from build123d import *

# Parameters (mm, degrees)
BOSS_EXTRU_1_DEPTH      = 21
ENL_V_MAT_EXTRU_1_REACH = 33.267
ESQUISSE2_R             = 3
ESQUISSE3_R             = 6
ENL_V_MAT_EXTRU_2_DEPTH = 10


with BuildPart() as part:
    # Esquisse1 → Boss.-Extru.1 (new body)
    with BuildSketch(Plane(origin=(0, 0, 0), x_dir=(0, 0, -1), z_dir=(1, 0, 0))):
        with BuildLine():
            Line((-42, -117.732748205), (-42, -149))
            Line((-42, -149), (42, -149))
            Line((42, -149), (42, -117.732748205))
            ThreePointArc((42, -117.732748205), (0, -125), (-42, -117.732748205))
        make_face()
    extrude(amount=BOSS_EXTRU_1_DEPTH)

    # Esquisse2 → Enlèv. mat.-Extru.1 (cut, up to next)
    with BuildSketch(Plane.XZ.offset(149), mode=Mode.PRIVATE) as enl_v_mat_extru_1_sk1:
        with Locations((10.5, 0)):
            Circle(ESQUISSE2_R)
    enl_v_mat_extru_1_tool1 = extrude(enl_v_mat_extru_1_sk1.sketch, amount=-ENL_V_MAT_EXTRU_1_REACH, mode=Mode.PRIVATE) & part.part
    add(enl_v_mat_extru_1_tool1.solids().sort_by_distance((10.5, -149, 0))[0], mode=Mode.SUBTRACT)

    # Esquisse3 → Enlèv. mat.-Extru.2 (cut)
    with BuildSketch(Plane.XZ.offset(149)):
        with Locations((10.560210211, 0)):
            Circle(ESQUISSE3_R)
    extrude(amount=-ENL_V_MAT_EXTRU_2_DEPTH, mode=Mode.SUBTRACT)


solid = part.part
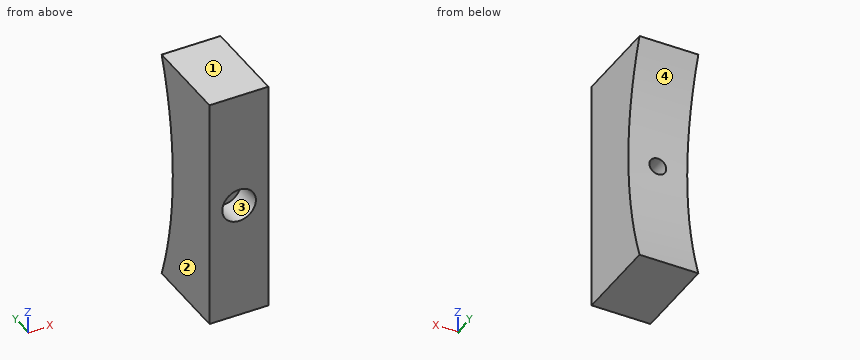
Geometry check sheet. Reference: the model listing, model coordinates, mm. Face numbers are marked on the shaded views. Give positions to 0.01 mm unless a question says otherwise; leave off trailing zeros. Order: outer loops, then holes, each group sorted by start corner. A loop starts at its lowest first (then second) coordinate and runs counter-clockwise, first axis right, second up. Notation, with made-up numbers: M -26.75,-19 L -15.75,-19 A11 ccw -15.75,-9 Z; hole C 20,25 d6. An arc over 180 degrees is marked long. Use a Markdown table: item, result.
Item 1: Section check D-D (x = 18.5). Record the cut outline in (y, z).
Answers follow:
| item | result |
|---|---|
| outline | M -149,-42 L -117.73,-42 A125 cw -117.73,42 L -149,42 Z |
Item 2: Material ranges on line 1 along X through (y, z) = (-131.75, 0); line 2 along Z through (x, y) = (10.5, -130.5); line 3 along Z through (x, y) = (13.75, -141.5), recorded low to high.
Answers follow:
| item | result |
|---|---|
| line 1 | x = 0 to 7.5, 13.5 to 21 |
| line 2 | z = -42 to -3, 3 to 42 |
| line 3 | z = -42 to -5.08, 5.08 to 42 |
Item 3: Section check B-B (x = 12). Record the cut outline in (y, z), and give its area (3 significant figures).
Answers follow:
| item | result |
|---|---|
| outline | M -149,-42 L -117.73,-42 A125 cw -124.97,-2.6 L -139,-2.6 L -139,-5.82 L -149,-5.82 Z; M -149,5.82 L -139,5.82 L -139,2.6 L -124.97,2.6 A125 cw -117.73,42 L -149,42 Z |
| area | 2,030 mm2 |
Item 4: Depth check by flat-ended pin: P1, Ø1, axis at x = 4.5, z = -18, coming from the +Y side; P2, Ø6, axis at x = 12.5, z = -2, coming from the -Y side; P3, Ø3, axis at x = 18.5, z = -1, coming from the +Y side (3 decimals); P4, Ø4, axis at y = -130.5, z = 16.5, coming from the -X side. Enter the tip coordinate at first touch or a pass-through.
Answers follow:
| item | result |
|---|---|
| P1 | stops at y = -123.62 |
| P2 | stops at y = -139 |
| P3 | stops at y = -124.975 |
| P4 | stops at x = 0 |
Item 5: Section check A-A (z = 0). Record the cut outline in (x, y).
Answers follow:
| item | result |
|---|---|
| outline | M 0,-149 L 4.56,-149 L 4.56,-139 L 7.5,-139 L 7.5,-125 L 0,-125 Z; M 13.5,-139 L 16.56,-139 L 16.56,-149 L 21,-149 L 21,-125 L 13.5,-125 Z |
Item 6: Draft check along Z on the marked faces 1, 2, 3 and 4. Enter one of: +Z half, -Z half, draft (parallel to the pull), parting line (faces both ways), or undercut.
Answers follow:
| item | result |
|---|---|
| face 1 | +Z half |
| face 2 | draft |
| face 3 | undercut |
| face 4 | undercut |
Item 7: Section check C-C (y = -137). Record the cut outline in (x, z).
Answers follow:
| item | result |
|---|---|
| outline | M 0,-42 L 21,-42 L 21,42 L 0,42 Z; hole C 10.5,0 d6 |
